Design review of the part built by this model. Coordinates are the model's own, in mm. Face numbers are marked on the shaded views. A direction names the side the tool comes from. Coordinates: 2 decimals unless noted, no trailing zeros. Write each loop counter-clockwise with the first axis right and the second up, starting at its lowest first coordinate (ties: lowest second). Pieces come first, ordered by that corner, then holes. Notation, with made-up numbers: (-6.75, 35.5) - (52.25, 35.5) arc R24 ccw to (52.25, 61.5) - close; hole circle Ø4 at (-8, 86). An arc over 180 degrees is marked (long way). Use a Markdown table: item, result.
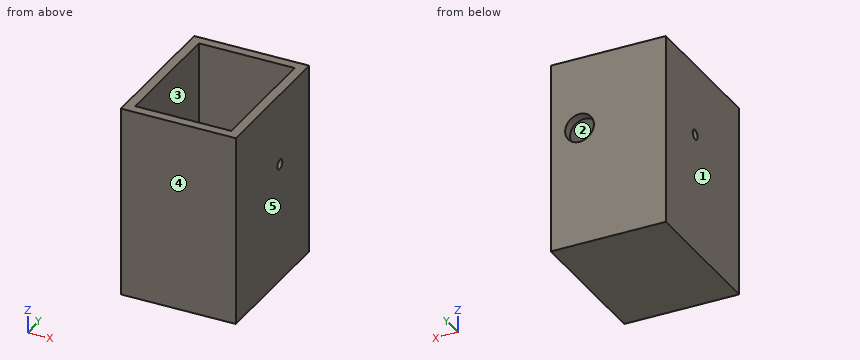
from build123d import *

# Parameters (mm, degrees)
SKETCH1_W           = 120
SKETCH1_H           = 150
BOSS_EXTRUDE1_DEPTH = 200
SKETCH2_W           = 100
SKETCH2_H           = 130
CUT_EXTRUDE1_DEPTH  = 195
SKETCH3_R           = 5
CUT_EXTRUDE2_DEPTH  = 120
CUT_EXTRUDE3_START  = -130
SKETCH4_R           = 15
CUT_EXTRUDE3_DEPTH  = 24


with BuildPart() as part:
    # Sketch1 → Boss-Extrude1 (new body)
    with BuildSketch(Plane.XY):
        with Locations((60, -75)):
            Rectangle(SKETCH1_W, SKETCH1_H)
    extrude(amount=BOSS_EXTRUDE1_DEPTH)

    # Sketch2 → Cut-Extrude1 (cut)
    with BuildSketch(Plane.XY.offset(200)):
        with Locations((60, -75)):
            Rectangle(SKETCH2_W, SKETCH2_H)
    extrude(amount=-CUT_EXTRUDE1_DEPTH, mode=Mode.SUBTRACT)

    # Sketch3 → Cut-Extrude2 (cut)
    with BuildSketch(Plane(origin=(120, 0, 0), x_dir=(0, 0, -1), z_dir=(1, 0, 0))):
        with Locations(Location((-125, -60, 0), (0, 0, 90))):
            Circle(SKETCH3_R)
    extrude(amount=-CUT_EXTRUDE2_DEPTH, mode=Mode.SUBTRACT)

    # Sketch4 → Cut-Extrude3 (cut)
    with BuildSketch(Plane.XZ.offset(150).offset(CUT_EXTRUDE3_START)):
        with Locations(Location((90, 125, 0), (0, 0, 270))):
            Circle(SKETCH4_R)
    extrude(amount=-CUT_EXTRUDE3_DEPTH, mode=Mode.SUBTRACT)


solid = part.part
(1) Take a section at A-A on y = -60. Write out the cut boundary in (x, z), and give its area (3 significant figures).
Determined:
| item | result |
|---|---|
| outline | (0, 0) - (120, 0) - (120, 120) - (110, 120) - (110, 5) - (10, 5) - (10, 120) - (0, 120) - close; (0, 130) - (10, 130) - (10, 200) - (0, 200) - close; (110, 130) - (120, 130) - (120, 200) - (110, 200) - close |
| area | 4,300 mm2 |
(2) Take a section at D-D on z = 50. Write out the cut boundary in (x, y), and give its area (3 significant figures).
Determined:
| item | result |
|---|---|
| outline | (0, -150) - (120, -150) - (120, 0) - (0, 0) - close; hole (10, -140) - (110, -140) - (110, -10) - (10, -10) - close |
| area | 5,000 mm2 |
(3) Take a section at B-B on z = 125. Write out the cut boundary in (x, y), and give its area (3 significant figures).
Determined:
| item | result |
|---|---|
| outline | (0, -150) - (120, -150) - (120, -65) - (110, -65) - (110, -140) - (10, -140) - (10, -65) - (0, -65) - close; (0, -55) - (10, -55) - (10, -10) - (75, -10) - (75, 0) - (0, 0) - close; (105, -10) - (110, -10) - (110, -55) - (120, -55) - (120, 0) - (105, 0) - close |
| area | 4,500 mm2 |
(4) For pin 1 (3 mm diameter, centred on x = 37.5, y = -92.5, fed in from +Z); pin 2 (1.5 mm diameter, centred on y = -84, z = 85.5, fed in from -X), all flat-tipped, find the tip position at first contact; note any pin that passes through.
Determined:
| item | result |
|---|---|
| pin 1 | z = 5 |
| pin 2 | x = 0 |
(5) Draft analysis for pull direction X (two halves, no side actions). For the marked faces 3, 4 and 5, state which applies: +X half, -X half, draft (parallel to the pull), parting line (faces both ways), or undercut.
Determined:
| item | result |
|---|---|
| face 3 | undercut |
| face 4 | draft |
| face 5 | +X half |
(6) Machinability: for the marked faces 1 and 2, which of the approach directions +Z, -Z, +X, -X, +Y, -Y give a long, thin tool a straight path to every point of the face, cutting with its end or side? Answer none if there is none.
Determined:
| item | result |
|---|---|
| face 1 | +Z, -Z, -X, +Y, -Y |
| face 2 | +Z |
(7) For L1, parallel to Y at x = 78, z = 137.5; L2, parallel to X at y = -136.5, z = 151; L3, parallel to X at y = -7.25, z = 125, list the stretches that pass through material, from the lowest coordinate up. Write a range as from..to.
Determined:
| item | result |
|---|---|
| L1 | -150..-140, -10..0 |
| L2 | 0..10, 110..120 |
| L3 | 0..75, 105..120 |
(8) Take a section at C-C on x = 81. Write out the cut boundary in (y, z).
Determined:
| item | result |
|---|---|
| outline | (-150, 0) - (0, 0) - (0, 113) - (-10, 113) - (-10, 5) - (-140, 5) - (-140, 200) - (-150, 200) - close; (-10, 137) - (0, 137) - (0, 200) - (-10, 200) - close |
